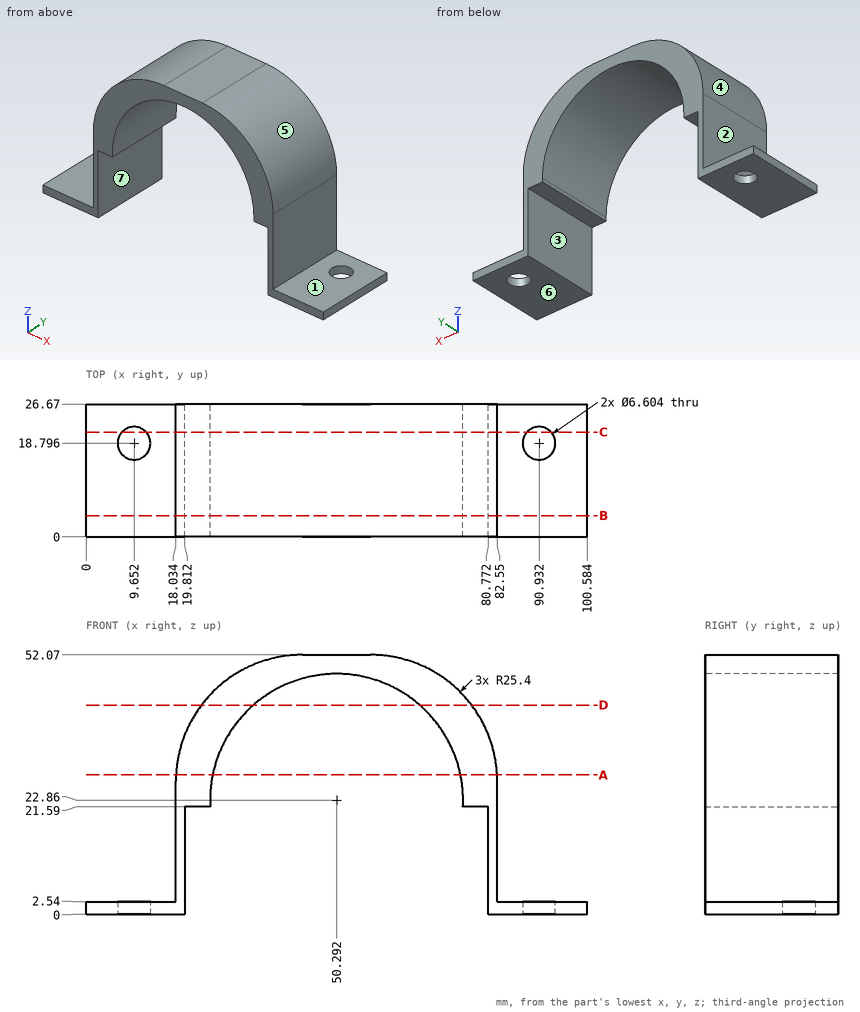
Verification items for this drawing (mm, ordinates from the low corner). A direction names the side the tool comes from. Round coordinates to 2 decimals unless told otherwise and drop trailing zeros. Write each loop counter-clockwise with the first axis right and the second up, starting at its lowest first coordinate (ties: lowest second). Pieces come first, ordered by that corner, then holes. Notation, with made-up numbers: (-6.5, 62.25) - (52.5, 62.25) arc R22 ccw to (52.5, 68.25) - close; hole circle Ø2 at (67.25, 68). An arc over 180 degrees is marked (long way). One line per item, written item: value.
1. Cross-section at A-A on z = 28. Record the boundary of the cut face in (x, y).
The answers:
outline: (18.07, 0) - (25.42, 0) - (25.42, 26.67) - (18.07, 26.67) - close; (75.17, 0) - (82.52, 0) - (82.52, 26.67) - (75.17, 26.67) - close
2. Scan lines: L1, parallel to X at y = 16.5, z = 21.5; L2, parallel to X at y = 19, z = 23; L3, parallel to Z at x = 14, y = 5.25. Record each from-to range of solid material in increasing order.
The answers:
L1: x = 18.03 to 19.81, 80.77 to 82.55
L2: x = 18.03 to 24.89, 75.69 to 82.55
L3: z = 0 to 2.54
3. Cross-section at C-C on y = 21. Record the boundary of the cut face in (x, z).
The answers:
outline: (0, 0) - (7.19, 0) - (7.19, 2.54) - (0, 2.54) - close; (12.11, 0) - (19.81, 0) - (19.81, 21.59) - (24.92, 21.59) arc R25.4 cw (long way) to (75.69, 22.86) arc R25.4 cw to (75.66, 21.59) - (80.77, 21.59) - (80.77, 0) - (88.47, 0) - (88.47, 2.54) - (82.55, 2.54) - (82.55, 26.67) arc R25.4 ccw to (57.15, 52.07) - (43.43, 52.07) arc R25.4 ccw to (18.03, 26.67) - (18.03, 2.54) - (12.11, 2.54) - close; (93.39, 0) - (100.58, 0) - (100.58, 2.54) - (93.39, 2.54) - close
4. Cross-section at D-D on z = 42. Record the boundary of the cut face in (x, y), and give its area (3 significant figures).
The answers:
outline: (23.18, 0) - (33.59, 0) - (33.59, 26.67) - (23.18, 26.67) - close; (66.99, 0) - (77.4, 0) - (77.4, 26.67) - (66.99, 26.67) - close
area: 555 mm^2
5. Mould release check, pull along X, two halves, no side actions. Record for the marked faces 4, 5, 6 and 7: released by +X, released by -X, zero draft, split by the parting line, or undercut.
The answers:
face 4: released by -X
face 5: released by +X
face 6: zero draft
face 7: undercut
6. Depth check by flat-ended pin: pin 1 Ø2.5 at (x, y) = (21.5, 9.5) entering from -Z; pin 2 Ø4 at (x, y) = (41, 12) entering from -Z; pin 3 Ø8 at (x, y) = (11.5, 9.5) entering from +Z. Enter the tip coordinate at first touch or a pass-through.
The answers:
pin 1: stops at z = 21.59
pin 2: stops at z = 45.61
pin 3: stops at z = 2.54
7. Set-up check for the marked faces 1, 2 and 3: record each of +Z, -Z, +X, -X, +Y, -Y from which the full face is reachable in a straight line by a thin tool's end or side.
The answers:
face 1: +Z, +X, +Y, -Y
face 2: +Z, -X, +Y, -Y
face 3: -Z, +Y, -Y
8. Cross-section at B-B on y = 4.25. Record the boundary of the cut face in (x, z).
The answers:
outline: (0, 0) - (19.81, 0) - (19.81, 21.59) - (24.92, 21.59) arc R25.4 cw (long way) to (75.69, 22.86) arc R25.4 cw to (75.66, 21.59) - (80.77, 21.59) - (80.77, 0) - (100.58, 0) - (100.58, 2.54) - (82.55, 2.54) - (82.55, 26.67) arc R25.4 ccw to (57.15, 52.07) - (43.43, 52.07) arc R25.4 ccw to (18.03, 26.67) - (18.03, 2.54) - (0, 2.54) - close
